Input: part model. Units: mm. Frame: model coordinates. Round coordinates to 2 decimals unless told otherwise and drop trailing zeros. Order: outer loops, then holes, each group sorted by start corner. A loop starts at its lowest first (then second) coordinate and runs counter-clockwise, first axis right, second up.
Item 1: Cut plane C-C on y = -48.5. Output: boundary loops of the cut face in (x, z), then the cut area to 3 significant figures.
Item 2: Cut plane A-A on y = -24.5. Output: boundary loops of the cut face in (x, z).
Item 3: Line query: L1, parallel to Y at x = 45, z = 0.65; L2, parallel to X at y = -88, z = 0.95; L3, parallel to X at y = -77, z = 0.3. Output: solid intervals per line, ascending.
Item 4: Cut plane B-B on z = 0.15. Output: boundary loops of the cut face in (x, y), then the cut area to 3 significant figures.
Item 5: First-contact query: pin 1 (0.5 mm diameter, centred on y = -95, z = 0.5, fed in from +X). Flat tip, straight axial feed; report the tip coordinate or a pass-through.
Item 6: Mould query, pull axis X, two halves, no side actions, for faces 1 (the cylindrical face through (46.433, -91.763, 0.493)), 2 (the flat face through (36, -64, 0)), 3 (the cylindrical face through (52.15, -126.99, 0.49)). Classes: released by +X, released by -X, zero draft, split by the parting line, or undercut.
```python
from build123d import *

# Parameters (mm, degrees)
SKETCH1_R           = 15
BOSS_EXTRUDE1_DEPTH = 1
CUT_EXTRUDE1_DEPTH  = 10


with BuildPart() as part:
    # Sketch1 → Boss-Extrude1 (new body)
    with BuildSketch(Plane(origin=(0, 0, 0), x_dir=(-1, 0, 0), z_dir=(0, 0, -1))):
        with BuildLine():
            Line((0, -75), (0, 0))
            Line((0, 0), (-90, 0))
            Line((-90, 0), (-90, -20))
            ThreePointArc((-90, -20), (-82.157527073, -45.383423367), (-61.363636364, -61.919344043))
            ThreePointArc((-61.363636364, -61.919344043), (-56.742771762, -65.593993082), (-55, -71.23475383))
            Line((-55, -71.23475383), (-55, -120))
            ThreePointArc((-55, -120), (-52.071067812, -127.071067812), (-45, -130))
            Line((-45, -130), (0, -130))
            Line((0, -130), (0, -75))
        make_face()
        with Locations((-45, -30)):
            Circle(SKETCH1_R, mode=Mode.SUBTRACT)
    extrude(amount=-BOSS_EXTRUDE1_DEPTH)

    # Sketch2 → Cut-Extrude1 (cut)
    with BuildSketch(Plane(origin=(0, 0, 0), x_dir=(-1, 0, 0), z_dir=(0, 0, -1))):
        with BuildLine():
            ThreePointArc((-43.646562299, -94.279689067), (-47.086223708, -91.795996374), (-49.569916401, -95.235657783))
            ThreePointArc((-49.569916401, -95.235657783), (-46.130254992, -97.719350476), (-43.646562299, -94.279689067))
        make_face()
        with BuildLine():
            ThreePointArc((-10.080889056, -88.862533012), (-6.641227647, -91.346225705), (-4.157534954, -87.906564297))
            ThreePointArc((-4.157534954, -87.906564297), (-7.597196363, -85.422871604), (-10.080889056, -88.862533012))
        make_face()
    extrude(amount=-CUT_EXTRUDE1_DEPTH, mode=Mode.SUBTRACT)


solid = part.part
```
From the geometry:
1. outline: (0, 0) - (79.82, 0) - (79.82, 1) - (0, 1) - close
1. area: 79.8 mm2
2. outline: (0, 0) - (31.04, 0) - (31.04, 1) - (0, 1) - close; (58.96, 0) - (89.77, 0) - (89.77, 1) - (58.96, 1) - close
3. L1: y = -130 to -97.29, -92.23 to -45, -15 to 0
3. L2: x = 0 to 4.14, 10.09 to 55
3. L3: x = 0 to 55
4. outline: (0, -130) - (45, -130) arc R10 ccw to (55, -120) - (55, -71.23) arc R10 cw to (61.36, -61.92) arc R45 ccw to (90, -20) - (90, 0) - (0, 0) - close; hole circle Ø6 at (7.12, -88.38); hole circle Ø30 at (45, -30); hole circle Ø6 at (46.61, -94.76)
4. area: 8,220 mm2
5. pin 1: stops at x = 55
6. face 1: undercut
6. face 2: zero draft
6. face 3: released by +X
